For this review, take the finished solid that the model builds, in its own axes (mm). Face numbers are marked on the shaded views. A direction names the side the tool comes from. Coordinates: 2 decimals unless noted, no trailing zeros. Loops run counter-clockwise (first coordinate to the right, second up) from the corner with the lowest first, then second, coordinate; pieces in that order, holes last.
1. Machinability: for the marked faces 4 and 5, which of the approach directions +Z, -Z, +X, -X, +Y, -Y give a long, thin tool a straight path to every point of the face, cutting with its end or side? Answer none if there is none.
2. Clearance check with flat-ended pins moving along their axes: P1, Ø3, axis at x = -18.5, z = 9, coming from the +Y side; P2, Ø12, axis at x = -2, z = 6, coming from the -Y side; P3, Ø5, axis at x = -30, z = 16, coming from the +Y side. State where each tip first meets the part, or that it passes through.
3. Take a section at B-B, the plane y = -39. State the section outline as (x, z) points, then the cut area to 3 significant figures.
4. To check wall thickness, follow probe 1 along Y at (x, z) = (-45.5, 3.75); probe 2 along Y at (x, z) = (-41.5, 4.75); probe 3 along X at (y, z) = (-18, 24). State the ranges of each line that lie inside material, in increasing order.
5. Mouldability with a two-part tool opening along Y and no side actions: class the marked faces 1, 2 and 3 as pulls with the +Y half, pulls with the -Y half, needs draft (parallel to the pull), parting line crosses it, or undercut.
6. Take a section at A-A, the plane x = 8. State the section outline as (y, z) points.
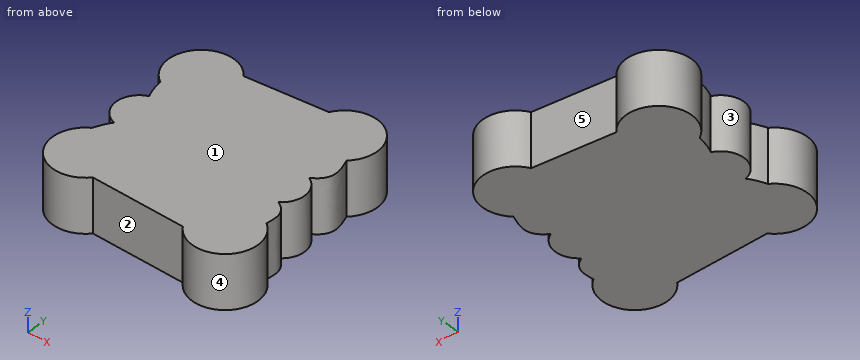
```python
from build123d import *

# Parameters (mm, degrees)
F1_DEPTH = 25.4


with BuildPart() as f1:
    # F0 (on Top) → F1 (new body)
    with BuildSketch(Plane.XY):
        with BuildLine():
            Line((15.3314765699, 45.3634702184), (-22.8350594245, 42.0886999699))
            ThreePointArc((-22.8350594245, 42.0886999699), (-46.5230995583, 43.1231755121), (-43.6973915181, 19.5815366758))
            add(Edge.make_bspline(
                [(-43.6973915181, 19.5815366758), (-43.1174367744, 16.2871292149), (-42.5374820306, 12.9927217539), (-41.0270827556, 10.2359403638)],
                knots=[0, 0, 0, 0, 0.3327137819, 0.3327137819, 0.3327137819, 0.3327137819], degree=3))
            add(Edge.make_bspline(
                [(-41.0270827556, 10.2359403638), (-40.5110375862, 9.2940545041), (-36.8442315299, 4.1334897017), (-28.1561256987, 1.87431405), (-20.9480811119, 0)],
                knots=[0.3327137819, 0.3327137819, 0.3327137819, 0.3327137819, 0.4463892469, 1, 1, 1, 1], degree=3))
            add(Edge.make_bspline(
                [(-40.1252666441, -10.5391209432), (-39.599730448, -9.8778116964), (-35.498491994, -5.4136644053), (-27.6646682205, -2.4989911865), (-20.9480811119, 0)],
                knots=[0.3384673734, 0.3384673734, 0.3384673734, 0.3384673734, 0.4328131906, 1, 1, 1, 1], degree=3))
            add(Edge.make_bspline(
                [(-44.2531548049, -18.2908964757), (-43.1318961623, -15.6012383193), (-42.0106375198, -12.911580163), (-40.1252666441, -10.5391209432)],
                knots=[0, 0, 0, 0, 0.3384673734, 0.3384673734, 0.3384673734, 0.3384673734], degree=3))
            ThreePointArc((-44.2531548049, -18.2908964757), (-47.768426214, -41.7394838947), (-24.0602315313, -41.4005297397))
            Line((-24.0602315313, -41.4005297397), (20.6953128024, -43.1810448239))
            ThreePointArc((20.6953128024, -43.1810448239), (44.3016536318, -45.4023187101), (42.6602594814, -21.7485830585))
            add(Edge.make_bspline(
                [(37.5745547292, -8.9566238299), (38.377714123, -9.423502034), (43.7248416865, -12.9867792586), (43.1537035595, -17.6874028342), (42.6602594814, -21.7485830585)],
                knots=[0.7611513259, 0.7611513259, 0.7611513259, 0.7611513259, 0.7936428016, 1, 1, 1, 1], degree=3))
            add(Edge.make_bspline(
                [(36.319540598, 9.7232166209), (30.2639633531, 5.8212058143), (11.0469761522, -0.50266664), (31.4704630142, -5.408302787), (37.5745547292, -8.9566238299)],
                knots=[0.2799466745, 0.2799466745, 0.2799466745, 0.2799466745, 0.5142128614, 0.7611513259, 0.7611513259, 0.7611513259, 0.7611513259], degree=3))
            add(Edge.make_bspline(
                [(39.7229749773, 26.7391821683), (41.6536861472, 21.6807257291), (44.0243403968, 15.4696199766), (37.6624586898, 10.5885479831), (36.319540598, 9.7232166209)],
                knots=[0, 0, 0, 0, 0.2279945174, 0.2799466745, 0.2799466745, 0.2799466745, 0.2799466745], degree=3))
            ThreePointArc((39.7229749773, 26.7391821683), (38.4970596178, 50.4180866311), (15.3314765699, 45.3634702184))
        make_face()
        with BuildLine():
            add(Edge.make_bspline(
                [(-41.0270827556, 10.2359403638), (-40.5110375862, 9.2940545041), (-36.8442315299, 4.1334897017), (-28.1561256987, 1.87431405), (-20.9480811119, 0)],
                knots=[0.3327137819, 0.3327137819, 0.3327137819, 0.3327137819, 0.4463892469, 1, 1, 1, 1], degree=3))
            ThreePointArc((-41.0270827556, 10.2359403638), (-48.0428369726, -0.4757075685), (-40.1252666441, -10.5391209432))
            add(Edge.make_bspline(
                [(-40.1252666441, -10.5391209432), (-39.599730448, -9.8778116964), (-35.498491994, -5.4136644053), (-27.6646682205, -2.4989911865), (-20.9480811119, 0)],
                knots=[0.3384673734, 0.3384673734, 0.3384673734, 0.3384673734, 0.4328131906, 1, 1, 1, 1], degree=3))
        make_face()
        with BuildLine():
            ThreePointArc((37.5745547292, -8.9566238299), (42.1864816242, 0.7353103047), (36.319540598, 9.7232166209))
            add(Edge.make_bspline(
                [(36.319540598, 9.7232166209), (30.2639633531, 5.8212058143), (11.0469761522, -0.50266664), (31.4704630142, -5.408302787), (37.5745547292, -8.9566238299)],
                knots=[0.2799466745, 0.2799466745, 0.2799466745, 0.2799466745, 0.5142128614, 0.7611513259, 0.7611513259, 0.7611513259, 0.7611513259], degree=3))
        make_face()
    extrude(amount=F1_DEPTH)


solid = f1.part
```
Results list:
1. face 4: +Z, -Z
1. face 5: +Z, -Z, +Y
2. P1: stops at y = 42.59
2. P2: stops at y = -42.52
2. P3: stops at y = 47.88
3. outline: (-49.68, 0) - (48.26, 0) - (48.26, 25.4) - (-49.68, 25.4) - close
3. area: 2,490 mm2
4. probe 1: y = -43.86 to -19.15, -7.04 to 7.04, 20.97 to 44.13
4. probe 2: y = -46.07 to -12.52, -10.04 to 10.04, 11.18 to 46.73
4. probe 3: x = -44.13 to 42.99
5. face 1: needs draft
5. face 2: pulls with the -Y half
5. face 3: undercut
6. outline: (-42.68, 0) - (44.73, 0) - (44.73, 25.4) - (-42.68, 25.4) - close
